```python
from build123d import *

# Parameters (mm, degrees)
F0_W     = 914.4
F0_H     = 406.4
F1_DEPTH = 9.525
F3_DEPTH = 406.4
F4_R     = 5


with BuildPart() as f1:
    # F0 (on Top) → F1 (new body)
    with BuildSketch(Plane.XY):
        Rectangle(F0_W, F0_H)
    extrude(amount=F1_DEPTH)

    # F2 (on face) → F3 (join, through all)
    with BuildSketch(Plane.XZ.offset(203.2)):
        with BuildLine():
            Line((-350.8375, 0), (-355.6, 0))
            Line((-355.6, 0), (-355.6, -45.8))
            ThreePointArc((-355.6, -45.8), (-354.135534, -49.335534), (-350.6, -50.8))
            Line((-350.6, -50.8), (-208.2, -50.8))
            ThreePointArc((-208.2, -50.8), (-204.664466, -49.335534), (-203.2, -45.8))
            Line((-203.2, -45.8), (-203.2, 0))
            Line((-203.2, 0), (-207.9625, 0))
            Line((-207.9625, 0), (-207.9625, -41.0375))
            ThreePointArc((-207.9625, -41.0375), (-209.426966, -44.573034), (-212.9625, -46.0375))
            Line((-212.9625, -46.0375), (-345.8375, -46.0375))
            ThreePointArc((-345.8375, -46.0375), (-349.373034, -44.573034), (-350.8375, -41.0375))
            Line((-350.8375, -41.0375), (-350.8375, 0))
        make_face()
        with BuildLine():
            Line((207.9625, 0), (203.2, 0))
            Line((203.2, 0), (203.2, -45.8))
            ThreePointArc((203.2, -45.8), (204.664466, -49.335534), (208.2, -50.8))
            Line((208.2, -50.8), (355.6, -50.8))
            Line((355.6, -50.8), (355.6, 0))
            Line((355.6, 0), (350.8375, 0))
            Line((350.8375, 0), (350.8375, -41.0375))
            ThreePointArc((350.8375, -41.0375), (349.373034, -44.573034), (345.8375, -46.0375))
            Line((345.8375, -46.0375), (212.9625, -46.0375))
            ThreePointArc((212.9625, -46.0375), (209.426966, -44.573034), (207.9625, -41.0375))
            Line((207.9625, -41.0375), (207.9625, 0))
        make_face()
    extrude(amount=-F3_DEPTH)

    # F4
    f4_edges = [f1.edges().sort_by_distance(p)[0] for p in [
        (355.6, 0, -50.8),
    ]]
    fillet(f4_edges, radius=F4_R)


solid = f1.part
```
The listing builds one solid part. Answer for the finished solid, in the listing's coordinates (mm). A direction names the side the tool comes from. Give positions to 0.01 mm unless a question says otherwise; leave off trailing zeros. Order: outer loops, then holes, each group sorted by start corner. A loop starts at its lowest first (then second) coordinate and runs counter-clockwise, first axis right, second up. Notation, with made-up numbers: (52, 6.25) - (94, 6.25) arc R34 cw to (94, 37.25) - close; hole circle Ø6 at (47, 2). An arc over 180 degrees is marked (long way). Use one line per item in the form item = value. Start each with the question number.
(1) For faces 1 (the flat face through (203.2, -3, -23)), 2 (the flat face through (-278, -3, -46.038)), 3 (the flat face through (406, 3, 0)), 4 (the flat face through (-407, 3, 0)), determine the directions among +Z, -Z, +X, -X, +Y, -Y from which every point of the face is accessible in a straight line to the end or side of a thin tool.
(2) The mould has two halves that part along Z. Classify faces 5 (the flat face through (-3, 3, 0)), 6 (the flat face through (355.6, -3, -23)), 7 (the flat face through (278, 3, 0)): released by +Z, released by -Z, zero draft, split by the parting line, or undercut.
(3) Consider line 1 (X direction, y = 53, z = -31.5); line 2 (Z direction, x = -239, y = 131) (1 decimal); line 3 (X direction, y = 108, z = -44). Determine where each line is inside the solid, lowest interval first. Write a range as from..to.
(4) A cutting plane is placed at B-B, the plane x = -231. Write down the section's boundary in (y, z) (1 decimal).
(5) A cutting plane is placed at A-A, the plane z = -18. Write down the section's boundary in (x, y), then the cut area to 3 significant figures.
(6) A cutting plane is placed at C-C, the plane y = 10. Write down the section's boundary in (x, z) (1 decimal).
(7) Flat-ended cylindrical pins translate along their axes: pin 1 Ø1 at (y, z) = (23.5, -28.5) entering from -X; pin 2 Ø12.5 at (y, z) = (-15.5, -17) entering from +X; pin 3 Ø1 at (x, y) = (172, -136.5) entering from -Z. Find the tip coordinate at first contact, or state that the pin passes through.
Ans:
q1.face_1 = -Z, +Y, -Y
q1.face_2 = +Y, -Y
q1.face_3 = -Z, +X, +Y, -Y
q1.face_4 = -Z, -X, +Y, -Y
q2.face_5 = released by -Z
q2.face_6 = zero draft
q2.face_7 = undercut
q3.line_1 = -355.6..-350.84, -207.96..-203.2, 203.2..207.96, 350.84..355.6
q3.line_2 = -50.8..-46, 0..9.5
q3.line_3 = -355.6..-349.87, -208.93..-203.2, 203.2..208.93, 349.87..355.6
q4.outline = (-203.2, -50.8) - (203.2, -50.8) - (203.2, -46) - (-203.2, -46) - close; (-203.2, 0) - (203.2, 0) - (203.2, 9.5) - (-203.2, 9.5) - close
q5.outline = (-355.6, -203.2) - (-350.84, -203.2) - (-350.84, 203.2) - (-355.6, 203.2) - close; (-207.96, -203.2) - (-203.2, -203.2) - (-203.2, 203.2) - (-207.96, 203.2) - close; (203.2, -203.2) - (207.96, -203.2) - (207.96, 203.2) - (203.2, 203.2) - close; (350.84, -203.2) - (355.6, -203.2) - (355.6, 203.2) - (350.84, 203.2) - close
q5.area = 7,740 mm^2
q6.outline = (-457.2, 0) - (-355.6, 0) - (-355.6, -45.8) arc R5 ccw to (-350.6, -50.8) - (-208.2, -50.8) arc R5 ccw to (-203.2, -45.8) - (-203.2, 0) - (203.2, 0) - (203.2, -45.8) arc R5 ccw to (208.2, -50.8) - (350.6, -50.8) arc R5 ccw to (355.6, -45.8) - (355.6, 0) - (457.2, 0) - (457.2, 9.5) - (-457.2, 9.5) - close; hole (-350.8, -41) arc R5 ccw to (-345.8, -46) - (-213, -46) arc R5 ccw to (-208, -41) - (-208, 0) - (-350.8, 0) - close; hole (208, -41) arc R5 ccw to (213, -46) - (345.8, -46) arc R5 ccw to (350.8, -41) - (350.8, 0) - (208, 0) - close
q7.pin_1 = -355.6
q7.pin_2 = 355.6
q7.pin_3 = 0
